```python
from build123d import *

# Parameters (mm, degrees)
SKETCH2_R           = 12.75
BOSS_EXTRUDE1_DEPTH = 56
SKETCH3_R           = 12.75
SKETCH3_R_2         = 3.25
BOSS_EXTRUDE2_DEPTH = 2


with BuildPart() as part:
    # Sketch2 → Boss-Extrude1 (new body)
    with BuildSketch(Plane(origin=(0, 0, 0), x_dir=(1, 0, 0), z_dir=(0, 1, 0))):
        with BuildLine():
            Line((-20, -16), (20, -16))
            Line((20, -16), (14.25, 0))
            ThreePointArc((14.25, 0), (0, 14.25), (-14.25, 0))
            Line((-14.25, 0), (-20, -16))
        make_face()
        with Locations(Location((0, 0, 0), (0, 0, 270))):
            Circle(SKETCH2_R, mode=Mode.SUBTRACT)
    extrude(amount=-BOSS_EXTRUDE1_DEPTH)

    # Sketch3 → Boss-Extrude2 (add)
    with BuildSketch(Plane(origin=(0, 0, 0), x_dir=(1, 0, 0), z_dir=(0, 1, 0))):
        with Locations(Location((0, 0, 0), (0, 0, 270))):
            Circle(SKETCH3_R)
        with Locations(Location((0, 0, 0), (0, 0, 270))):
            Circle(SKETCH3_R_2, mode=Mode.SUBTRACT)
    extrude(amount=-BOSS_EXTRUDE2_DEPTH)


solid = part.part
```
Source: CAD feature listing. Evaluate the final solid. Frame: model axes, mm. A direction names the side the tool comes from. Give positions to 0.01 mm unless a question says otherwise; leave off trailing zeros. Order: outer loops, then holes, each group sorted by start corner. A loop starts at its lowest first (then second) coordinate and runs counter-clockwise, first axis right, second up.
(1) Section query D-D (z = 9). Return the cut outline in (x, y), plus the area to 3 significant figures.
(2) Contact query for flat-ended pins moving along their axis: P1, Ø7.5, axis at x = -1.5, z = 5, coming from the -Y side; P2, Ø4, axis at y = -48.5, z = -1, coming from the -X side; P3, Ø8, axis at y = -34.5, z = 7.5, coming from the +X side. Output: stop coordinate, or through.
(3) Material intervals for line 1 along X through (y, z) = (-1, 0); line 2 along X through (y, z) = (-25, 0); line 3 along Y through (x, z) = (-6, -7), sorted ascending.
(4) Section query C-C (x = -7.5). Return the cut outline in (y, z), plus the area to 3 significant figures.
(5) Section query B-B (y = -5.5). Return the cut outline in (x, z), plus the area to 3 significant figures.
(6) Section query A-A (x = 0). Return the cut outline in (y, z).
(7) Pull-direction query (X, two-part tool) for faces 3 (the face through (0.313, -27.608, -14.247)), 4 (the face through (-12.447, -28.622, -2.764)), 5 (the face through (-17.085, -27.608, 7.888)); classes: +X half, -X half, draft (parallel to the pull), parting line (faces both ways), or undercut.
(8) Access query for faces 1 (the face through (-1.978, -0.986, -2.579)), 2 (the face through (-3, -2, 3)). Directions: +Z, -Z, +X, -X, +Y, -Y. A direction counts if a zero-diameter tool reaches every point of the face in a straight line with its end or side. Return the directions, or none.
Outcome:
1. outline: (-17.48, -56) - (-9.03, -56) - (-9.03, -2) - (9.03, -2) - (9.03, -56) - (17.48, -56) - (17.48, 0) - (-17.48, 0) - close
1. area: 983 mm2
2. P1: stops at y = -2
2. P2: stops at x = -14.61
2. P3: stops at x = 18.38
3. line 1: x = -14.25 to -3.25, 3.25 to 14.25
3. line 2: x = -14.25 to -12.75, 12.75 to 14.25
3. line 3: y = -2 to 0
4. outline: (-56, -12.12) - (0, -12.12) - (0, 16) - (-56, 16) - (-56, 10.31) - (-2, 10.31) - (-2, -10.31) - (-56, -10.31) - close
4. area: 461 mm2
5. outline: (-20, 16) - (-14.25, 0) arc R14.25 ccw to (14.25, 0) - (20, 16) - close; hole circle Ø25.5 at (0, 0)
5. area: 356 mm2
6. outline: (-56, -14.25) - (0, -14.25) - (0, -3.25) - (-2, -3.25) - (-2, -12.75) - (-56, -12.75) - close; (-56, 12.75) - (-2, 12.75) - (-2, 3.25) - (0, 3.25) - (0, 16) - (-56, 16) - close
7. face 3: parting line
7. face 4: undercut
7. face 5: -X half
8. face 1: +Y, -Y
8. face 2: -Y
